Could you check a few things on this model? Use its own coordinates, in mm. A direction names the side the tool comes from. Give positions to 0.01 mm unless a question says otherwise; leave off trailing zeros. Order: outer loops, then holes, each group sorted by start corner. A loop starts at its lowest first (then second) coordinate and runs counter-clockwise, first axis right, second up. Notation, with made-up numbers: (63, -28) -> (91, -28) arc R23 cw to (91, 1) -> close; hole circle Ø6 at (40.5, 72.25). An arc over 180 degrees is marked (long way). Answer as CSV lines item,"result". Start each with the question number.
(1) I want a section at C-C (z = 20.5). Give the number of separate pieces and of enclosed holes in the cut face, plus the area to 3 significant figures.
(2) I need wall thicknesses on L1, parallel to Y at x = -11.6, z = 67.5; L2, parallel to X at y = 4.5, z = 44.5; L3, parallel to Y at x = 0, z = 65. Which ranges of each line are inside material? Lowest first, please.
(3) We'd pull the mould along Y, two halves only. Please class faces 1 (the face through (69, 15, 49)), 2 (the face through (6, 0, 49)), 3 (the face through (15, -15, 49)): released by +Y, released by -Y, zero draft, split by the parting line, or undercut.
(4) I want a section at B-B (y = 0). Please give me the cut outline in (x, z).
(5) I want a section at A-A (x = 30). Please give me the cut outline in (y, z).
(6) On a 3-axis mill with a long thin cutter (end or side, diameter ignored), from which of +Z, -Z, +X, -X, +Y, -Y can I reach the whole of each face in a straight line? I mean faces 4 (the face through (69, -15, 49)), 5 (the face through (68.25, 11, 49)). Say none if no direction works.
(7) Will these pins go through, and if not, where does the flat tip stop? pin 1 Ø4.5 at (y, z) = (1.5, 47) entering from +X; pin 2 Ø0.8 at (y, z) = (-14, 57) entering from +X; pin 3 Ø2 at (y, z) = (-2.5, 38) entering from -X.
```python
from build123d import *

# Parameters (mm, degrees)
SKETCH_1_R      = 3.4
SKETCH_1_R_2    = 2.1
EXTRUDE_1_DEPTH = 100


with BuildPart() as part:
    # 草图1 → 凸台-拉伸1 (new body)
    with BuildSketch(Plane.XY):
        with BuildLine():
            Line((-15, 13), (-15, 4.3))
            ThreePointArc((-15, 4.3), (-14.912132034, 4.087867966), (-14.7, 4))
            Line((-14.7, 4), (-13, 4))
            Line((-13, 4), (-13, 8.25))
            Line((-13, 8.25), (-9.664213562, 8.25))
            Line((-9.664213562, 8.25), (-6, 4.585786438))
            Line((-6, 4.585786438), (-6, -4.585786438))
            Line((-6, -4.585786438), (-9.664213562, -8.25))
            Line((-9.664213562, -8.25), (-13, -8.25))
            Line((-13, -8.25), (-13, -4))
            Line((-13, -4), (-14.7, -4))
            ThreePointArc((-14.7, -4), (-14.912132034, -4.087867966), (-15, -4.3))
            Line((-15, -4.3), (-15, -13))
            ThreePointArc((-15, -13), (-14.414213562, -14.414213562), (-13, -15))
            Line((-13, -15), (-4.3, -15))
            ThreePointArc((-4.3, -15), (-4.087867966, -14.912132034), (-4, -14.7))
            Line((-4, -14.7), (-4, -13))
            Line((-4, -13), (-8.25, -13))
            Line((-8.25, -13), (-8.25, -9.664213562))
            Line((-8.25, -9.664213562), (-4.585786438, -6))
            Line((-4.585786438, -6), (4.585786438, -6))
            Line((4.585786438, -6), (8.25, -9.664213562))
            Line((8.25, -9.664213562), (8.25, -13))
            Line((8.25, -13), (4, -13))
            Line((4, -13), (4, -14.7))
            ThreePointArc((4, -14.7), (4.087867966, -14.912132034), (4.3, -15))
            Line((4.3, -15), (25.7, -15))
            ThreePointArc((25.7, -15), (25.912132034, -14.912132034), (26, -14.7))
            Line((26, -14.7), (26, -13))
            Line((26, -13), (21.75, -13))
            Line((21.75, -13), (21.75, -9.664213562))
            Line((21.75, -9.664213562), (25.414213562, -6))
            Line((25.414213562, -6), (34.585786438, -6))
            Line((34.585786438, -6), (38.25, -9.664213562))
            Line((38.25, -9.664213562), (38.25, -13))
            Line((38.25, -13), (34, -13))
            Line((34, -13), (34, -14.7))
            ThreePointArc((34, -14.7), (34.087867966, -14.912132034), (34.3, -15))
            Line((34.3, -15), (55.7, -15))
            ThreePointArc((55.7, -15), (55.912132034, -14.912132034), (56, -14.7))
            Line((56, -14.7), (56, -13))
            Line((56, -13), (51.75, -13))
            Line((51.75, -13), (51.75, -9.664213562))
            Line((51.75, -9.664213562), (55.414213562, -6))
            Line((55.414213562, -6), (64.585786438, -6))
            Line((64.585786438, -6), (68.25, -9.664213562))
            Line((68.25, -9.664213562), (68.25, -13))
            Line((68.25, -13), (64, -13))
            Line((64, -13), (64, -14.7))
            ThreePointArc((64, -14.7), (64.087867966, -14.912132034), (64.3, -15))
            Line((64.3, -15), (73, -15))
            ThreePointArc((73, -15), (74.414213562, -14.414213562), (75, -13))
            Line((75, -13), (75, -4.3))
            ThreePointArc((75, -4.3), (74.912132034, -4.087867966), (74.7, -4))
            Line((74.7, -4), (73, -4))
            Line((73, -4), (73, -8.25))
            Line((73, -8.25), (69.664213562, -8.25))
            Line((69.664213562, -8.25), (66, -4.585786438))
            Line((66, -4.585786438), (66, 4.585786438))
            Line((66, 4.585786438), (69.664213562, 8.25))
            Line((69.664213562, 8.25), (73, 8.25))
            Line((73, 8.25), (73, 4))
            Line((73, 4), (74.7, 4))
            ThreePointArc((74.7, 4), (74.912132034, 4.087867966), (75, 4.3))
            Line((75, 4.3), (75, 13))
            ThreePointArc((75, 13), (74.414213562, 14.414213562), (73, 15))
            Line((73, 15), (64.3, 15))
            ThreePointArc((64.3, 15), (64.087867966, 14.912132034), (64, 14.7))
            Line((64, 14.7), (64, 13))
            Line((64, 13), (68.25, 13))
            Line((68.25, 13), (68.25, 9.664213562))
            Line((68.25, 9.664213562), (64.585786438, 6))
            Line((64.585786438, 6), (55.414213562, 6))
            Line((55.414213562, 6), (51.75, 9.664213562))
            Line((51.75, 9.664213562), (51.75, 13))
            Line((51.75, 13), (56, 13))
            Line((56, 13), (56, 14.7))
            ThreePointArc((56, 14.7), (55.912132034, 14.912132034), (55.7, 15))
            Line((55.7, 15), (34.3, 15))
            ThreePointArc((34.3, 15), (34.087867966, 14.912132034), (34, 14.7))
            Line((34, 14.7), (34, 13))
            Line((34, 13), (38.25, 13))
            Line((38.25, 13), (38.25, 9.664213562))
            Line((38.25, 9.664213562), (34.585786438, 6))
            Line((34.585786438, 6), (25.414213562, 6))
            Line((25.414213562, 6), (21.75, 9.664213562))
            Line((21.75, 9.664213562), (21.75, 13))
            Line((21.75, 13), (26, 13))
            Line((26, 13), (26, 14.7))
            ThreePointArc((26, 14.7), (25.912132034, 14.912132034), (25.7, 15))
            Line((25.7, 15), (4.3, 15))
            ThreePointArc((4.3, 15), (4.087867966, 14.912132034), (4, 14.7))
            Line((4, 14.7), (4, 13))
            Line((4, 13), (8.25, 13))
            Line((8.25, 13), (8.25, 9.664213562))
            Line((8.25, 9.664213562), (4.585786438, 6))
            Line((4.585786438, 6), (-4.585786438, 6))
            Line((-4.585786438, 6), (-8.25, 9.664213562))
            Line((-8.25, 9.664213562), (-8.25, 13))
            Line((-8.25, 13), (-4, 13))
            Line((-4, 13), (-4, 14.7))
            ThreePointArc((-4, 14.7), (-4.087867966, 14.912132034), (-4.3, 15))
            Line((-4.3, 15), (-13, 15))
            ThreePointArc((-13, 15), (-14.414213562, 14.414213562), (-15, 13))
        make_face()
        Circle(SKETCH_1_R, mode=Mode.SUBTRACT)
        with Locations((60, 0)):
            Circle(SKETCH_1_R, mode=Mode.SUBTRACT)
        with Locations((30, 0)):
            Circle(SKETCH_1_R, mode=Mode.SUBTRACT)
        with Locations((-11.6, -11.65)):
            Circle(SKETCH_1_R_2, mode=Mode.SUBTRACT)
        with Locations((71.6, -11.65)):
            Circle(SKETCH_1_R_2, mode=Mode.SUBTRACT)
        with Locations((71.6, 11.65)):
            Circle(SKETCH_1_R_2, mode=Mode.SUBTRACT)
        with Locations((-11.6, 11.65)):
            Circle(SKETCH_1_R_2, mode=Mode.SUBTRACT)
        with BuildLine():
            Line((40.25, 11), (40.25, 10))
            Line((40.25, 10), (40.25, 8.835786438))
            Line((40.25, 8.835786438), (36, 4.585786438))
            Line((36, 4.585786438), (36, -4.585786438))
            Line((36, -4.585786438), (40.25, -8.835786438))
            Line((40.25, -8.835786438), (40.25, -10))
            Line((40.25, -10), (40.25, -11))
            ThreePointArc((40.25, -11), (40.542893219, -11.707106781), (41.25, -12))
            Line((41.25, -12), (48.75, -12))
            ThreePointArc((48.75, -12), (49.457106781, -11.707106781), (49.75, -11))
            Line((49.75, -11), (49.75, -10))
            Line((49.75, -10), (49.75, -8.835786438))
            Line((49.75, -8.835786438), (54, -4.585786438))
            Line((54, -4.585786438), (54, 4.585786438))
            Line((54, 4.585786438), (49.75, 8.835786438))
            Line((49.75, 8.835786438), (49.75, 10))
            Line((49.75, 10), (49.75, 11))
            ThreePointArc((49.75, 11), (49.457106781, 11.707106781), (48.75, 12))
            Line((48.75, 12), (41.25, 12))
            ThreePointArc((41.25, 12), (40.542893219, 11.707106781), (40.25, 11))
        make_face(mode=Mode.SUBTRACT)
        with BuildLine():
            Line((18.75, 12), (11.25, 12))
            ThreePointArc((11.25, 12), (10.542893219, 11.707106781), (10.25, 11))
            Line((10.25, 11), (10.25, 10))
            Line((10.25, 10), (10.25, 8.835786438))
            Line((10.25, 8.835786438), (6, 4.585786438))
            Line((6, 4.585786438), (6, -4.585786438))
            Line((6, -4.585786438), (10.25, -8.835786438))
            Line((10.25, -8.835786438), (10.25, -10))
            Line((10.25, -10), (10.25, -11))
            ThreePointArc((10.25, -11), (10.542893219, -11.707106781), (11.25, -12))
            Line((11.25, -12), (18.75, -12))
            ThreePointArc((18.75, -12), (19.457106781, -11.707106781), (19.75, -11))
            Line((19.75, -11), (19.75, -10))
            Line((19.75, -10), (19.75, -8.835786438))
            Line((19.75, -8.835786438), (24, -4.585786438))
            Line((24, -4.585786438), (24, 4.585786438))
            Line((24, 4.585786438), (19.75, 8.835786438))
            Line((19.75, 8.835786438), (19.75, 10))
            Line((19.75, 10), (19.75, 11))
            ThreePointArc((19.75, 11), (19.457106781, 11.707106781), (18.75, 12))
        make_face(mode=Mode.SUBTRACT)
    extrude(amount=EXTRUDE_1_DEPTH)


solid = part.part
```
Final values:
1,separate pieces,"1"
1,enclosed holes,"9"
1,area,"905 mm²"
2,L1,"-15 to -13.75, -9.55 to -8.25, 8.25 to 9.55, 13.75 to 15"
2,L2,"-15 to -13, -6 to 6, 24 to 36, 54 to 66, 73 to 75"
2,L3,"-6 to -3.4, 3.4 to 6"
3,face 1,"released by +Y"
3,face 2,"undercut"
3,face 3,"released by -Y"
4,outline,"(-6, 0) -> (-3.4, 0) -> (-3.4, 100) -> (-6, 100) -> close; (3.4, 0) -> (6, 0) -> (6, 100) -> (3.4, 100) -> close; (24, 0) -> (26.6, 0) -> (26.6, 100) -> (24, 100) -> close; (33.4, 0) -> (36, 0) -> (36, 100) -> (33.4, 100) -> close; (54, 0) -> (56.6, 0) -> (56.6, 100) -> (54, 100) -> close; (63.4, 0) -> (66, 0) -> (66, 100) -> (63.4, 100) -> close"
5,outline,"(-6, 0) -> (-3.4, 0) -> (-3.4, 100) -> (-6, 100) -> close; (3.4, 0) -> (6, 0) -> (6, 100) -> (3.4, 100) -> close"
6,face 4,"+Z, -Z, +X, -X, -Y"
6,face 5,"+Z, -Z"
7,pin 1,"x = 66"
7,pin 2,"x = 74.91"
7,pin 3,"x = -6"
